from build123d import *

# Parameters (mm, degrees)
SKETCH1_W           = 180.975
SKETCH1_H           = 50.8
SKETCH1_W_2         = 26.9875
SKETCH1_H_2         = 26.9875
BOSS_EXTRUDE1_DEPTH = 6.35
SKETCH3_R           = 3.175
BOSS_EXTRUDE2_DEPTH = 101.6
SKETCH4_R           = 12.7
BOSS_EXTRUDE3_DEPTH = 50.8


with BuildPart() as part:
    # Sketch1 → Boss-Extrude1 (new body)
    with BuildSketch(Plane(origin=(0, 0, 0), x_dir=(1, 0, 0), z_dir=(0, 1, 0))):
        with Locations((-90.4875, -25.4)):
            Rectangle(SKETCH1_W, SKETCH1_H)
        with Locations((-162.71875, -25.4)):
            Rectangle(SKETCH1_W_2, SKETCH1_H_2, mode=Mode.SUBTRACT)
        with Locations((-18.25625, -25.4)):
            Rectangle(SKETCH1_W_2, SKETCH1_H_2, mode=Mode.SUBTRACT)
    extrude(amount=BOSS_EXTRUDE1_DEPTH)

    # Sketch3 → Boss-Extrude2 (add)
    with BuildSketch(Plane(origin=(0, 6.35, 0), x_dir=(1, 0, 0), z_dir=(0, 1, 0))):
        with Locations(Location((-77.7875, -38.1, 0), (0, 0, 90))):
            Circle(SKETCH3_R)
        with Locations(Location((-103.1875, -12.7, 0), (0, 0, 90))):
            Circle(SKETCH3_R)
    extrude(amount=BOSS_EXTRUDE2_DEPTH)

    # Sketch4 → Boss-Extrude3 (add)
    with BuildSketch(Plane(origin=(0, 6.35, 0), x_dir=(1, 0, 0), z_dir=(0, 1, 0))):
        with Locations(Location((-103.1875, -12.7, 0), (0, 0, 90))):
            Circle(SKETCH4_R)
        with Locations(Location((-77.7875, -38.1, 0), (0, 0, 270))):
            Circle(SKETCH4_R)
    extrude(amount=BOSS_EXTRUDE3_DEPTH)


solid = part.part
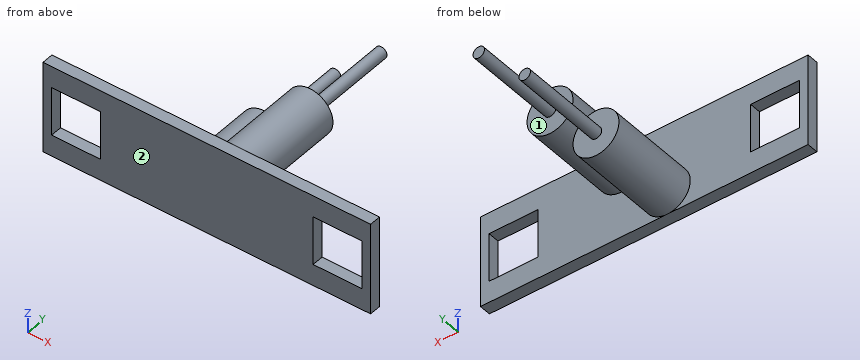
Part model, mm, in its own coordinate system. Face numbers are marked on the shaded views. A direction names the side the tool comes from. Give positions to 0.01 mm unless a question says otherwise; leave off trailing zeros. Order: outer loops, then holes, each group sorted by start corner. A loop starts at its lowest first (then second) coordinate and runs counter-clockwise, first axis right, second up. Notation, with made-up numbers: (25, -11.5) - (58, -11.5) arc R27 ccw to (58, 5.5) - close; hole circle Ø3 at (-28, -19). An arc over 180 degrees is marked (long way). Use a Markdown table: item, result.
1) 3-axis set-ups, long thin cutter, end or side, ignore diameter. For the marked faces 1 and 2: which of +Z, -Z, +X, -X, +Y, -Y reach the whole face in a straight line?
Checked values:
| item | result |
|---|---|
| face 1 | +Y |
| face 2 | +Z, -Z, +X, -X, -Y |
2) Probe L1, parallel to Y at x = -123.5, z = 43.5; L2, parallel to X at y = 43, z = 12; L3, parallel to Z at x = -103, y = 63.5. List the from-to ranges inside material, lowest first. Write a range as from..to.
Checked values:
| item | result |
|---|---|
| L1 | 0..6.35 |
| L2 | -115.87..-90.51 |
| L3 | 9.53..15.87 |
3) Saw through at D-D on x = -72. List the corners of the cut face in (y, z).
Checked values:
| item | result |
|---|---|
| outline | (0, 0) - (6.35, 0) - (6.35, 26.8) - (57.15, 26.8) - (57.15, 49.4) - (6.35, 49.4) - (6.35, 50.8) - (0, 50.8) - close |
4) Saw through at C-C on z = 45. List the corners of the cut face in (x, y) (3 decimals), plus the area to 3 significant figures.
Checked values:
| item | result |
|---|---|
| outline | (-180.975, 0) - (0, 0) - (0, 6.35) - (-67.125, 6.35) - (-67.125, 57.15) - (-88.45, 57.15) - (-88.45, 6.35) - (-180.975, 6.35) - close |
| area | 2,230 mm² |
5) Saw through at A-A on x = -26. List the corners of the cut face in (y, z), plus the area to 3 significant figures.
Checked values:
| item | result |
|---|---|
| outline | (0, 0) - (6.35, 0) - (6.35, 11.91) - (0, 11.91) - close; (0, 38.89) - (6.35, 38.89) - (6.35, 50.8) - (0, 50.8) - close |
| area | 151 mm² |
6) Saw through at B-B on z = 21.5. Count the separate pieces of the cut face and the enclosed holes in it, plus the area to 3 significant figures.
Checked values:
| item | result |
|---|---|
| separate pieces | 3 |
| enclosed holes | 0 |
| area | 1,740 mm² |
7) Flat gauge pins, fed straight in: P1, Ø10, axis at y = 72.5, z = 29, coming from the -X side; P2, Ø12, axis at y = 16.5, z = 31.5, coming from the +X side; P3, Ø3, axis at y = 2.5, z = 21, coming from the +X side; P4, Ø1, axis at x = -59, z = 26, coming from the +Y side. Where does each tip first touch, or does it go through?
Checked values:
| item | result |
|---|---|
| P1 | through |
| P2 | x = -65.1 |
| P3 | x = 0 |
| P4 | y = 6.35 |
